```python
from build123d import *

# Parameters (mm, degrees)
SKETCH1_R           = 30
SKETCH1_R_2         = 21
BOSS_EXTRUDE1_DEPTH = 14
SKETCH1_3_R         = 32.5
SKETCH1_3_R_2       = 30
SKETCH1_3_R_3       = 21
BOSS_EXTRUDE2_DEPTH = 42
CUT_EXTRUDE1_START  = 14
SKETCH1_4_R         = 32.5
SKETCH1_4_R_2       = 30
CUT_EXTRUDE1_DEPTH  = 3
CHAMFER2_SIZE       = 2


with BuildPart() as part:
    # Sketch1 → Boss-Extrude1 (new body)
    # profile 1 of 8: a face of its own
    with BuildSketch(Plane(origin=(0, 0, 0), x_dir=(1, 0, 0), z_dir=(0, 1, 0))):
        Polygon((-18.763883749, -32.5), (18.763883749, -32.5), (37.527767497, 0), (18.763883749, 32.5), (-18.763883749, 32.5), (-37.527767497, 0), align=None)
        Circle(SKETCH1_R, mode=Mode.SUBTRACT)
    # profile 2 of 8: a face of its own
    with BuildSketch(Plane(origin=(0, 0, 0), x_dir=(1, 0, 0), z_dir=(0, 1, 0))):
        Circle(SKETCH1_R)
        with Locations(Location((0, 0, 0), (0, 0, 270))):
            Circle(SKETCH1_R_2, mode=Mode.SUBTRACT)
    # profile 3 of 8: a face of its own
    with BuildSketch(Plane(origin=(0, 0, 0), x_dir=(1, 0, 0), z_dir=(0, 1, 0))):
        with BuildLine():
            ThreePointArc((-5.3e-08, 32.5), (16.250000065, 28.145825585), (28.145825725, 16.249999824))
            Line((28.145825725, 16.249999824), (18.763883749, 32.5))
            Line((18.763883749, 32.5), (-5.3e-08, 32.5))
        make_face()
    # profile 4 of 8: a face of its own
    with BuildSketch(Plane(origin=(0, 0, 0), x_dir=(1, 0, 0), z_dir=(0, 1, 0))):
        with BuildLine():
            ThreePointArc((-28.14582555, 16.250000126), (-16.24999996, 28.145825646), (-5.3e-08, 32.5))
            Line((-5.3e-08, 32.5), (-18.763883749, 32.5))
            Line((-18.763883749, 32.5), (-28.14582555, 16.250000126))
        make_face()
    # profile 5 of 8: a face of its own
    with BuildSketch(Plane(origin=(0, 0, 0), x_dir=(1, 0, 0), z_dir=(0, 1, 0))):
        with BuildLine():
            Line((28.145825318, -16.250000528), (37.527767497, 0))
            Line((37.527767497, 0), (28.145825725, 16.249999824))
            ThreePointArc((28.145825725, 16.249999824), (31.392589381, 8.411618868), (32.5, 0))
            ThreePointArc((32.5, 0), (31.392589275, -8.41161926), (28.145825318, -16.250000528))
        make_face()
    # profile 6 of 8: a face of its own
    with BuildSketch(Plane(origin=(0, 0, 0), x_dir=(1, 0, 0), z_dir=(0, 1, 0))):
        with BuildLine():
            Line((18.763883749, -32.5), (28.145825318, -16.250000528))
            ThreePointArc((28.145825318, -16.250000528), (16.249999715, -28.145825788), (-4.8e-08, -32.5))
            Line((-4.8e-08, -32.5), (18.763883749, -32.5))
        make_face()
    # profile 7 of 8: a face of its own
    with BuildSketch(Plane(origin=(0, 0, 0), x_dir=(1, 0, 0), z_dir=(0, 1, 0))):
        with BuildLine():
            Line((-18.763883749, -32.5), (-4.8e-08, -32.5))
            ThreePointArc((-4.8e-08, -32.5), (-16.250000055, -28.145825591), (-28.145825663, -16.249999931))
            Line((-28.145825663, -16.249999931), (-18.763883749, -32.5))
        make_face()
    # profile 8 of 8: a face of its own
    with BuildSketch(Plane(origin=(0, 0, 0), x_dir=(1, 0, 0), z_dir=(0, 1, 0))):
        with BuildLine():
            ThreePointArc((-28.145825663, -16.249999931), (-32.5, 1.12e-07), (-28.14582555, 16.250000126))
            Line((-28.14582555, 16.250000126), (-37.527767497, 0))
            Line((-37.527767497, 0), (-28.145825663, -16.249999931))
        make_face()
    extrude(amount=BOSS_EXTRUDE1_DEPTH)

    # Sketch1<3> → Boss-Extrude2 (add)
    # profile 1 of 2: a face of its own
    with BuildSketch(Plane(origin=(0, 0, 0), x_dir=(1, 0, 0), z_dir=(0, 1, 0))):
        with Locations(Location((0, 0, 0), (0, 0, 270))):
            Circle(SKETCH1_3_R)
        Circle(SKETCH1_3_R_2, mode=Mode.SUBTRACT)
    # profile 2 of 2: a face of its own
    with BuildSketch(Plane(origin=(0, 0, 0), x_dir=(1, 0, 0), z_dir=(0, 1, 0))):
        Circle(SKETCH1_3_R_2)
        with Locations(Location((0, 0, 0), (0, 0, 270))):
            Circle(SKETCH1_3_R_3, mode=Mode.SUBTRACT)
    extrude(amount=BOSS_EXTRUDE2_DEPTH)

    # Sketch1<4> → Cut-Extrude1 (cut)
    with BuildSketch(Plane(origin=(0, 0, 0), x_dir=(1, 0, 0), z_dir=(0, 1, 0)).offset(CUT_EXTRUDE1_START)):
        with Locations(Location((0, 0, 0), (0, 0, 90))):
            Circle(SKETCH1_4_R)
        with Locations(Location((0, 0, 0), (0, 0, 270))):
            Circle(SKETCH1_4_R_2, mode=Mode.SUBTRACT)
    extrude(amount=CUT_EXTRUDE1_DEPTH, mode=Mode.SUBTRACT)

    # Chamfer2
    chamfer2_edges = [part.edges().sort_by_distance(p)[0] for p in [
        (0, 42, -32.5),
    ]]
    chamfer(chamfer2_edges, length=CHAMFER2_SIZE)


solid = part.part
```
Part model, mm, in its own coordinate system. A direction names the side the tool comes from. Coordinates: 2 decimals unless noted, no trailing zeros. Order: outer loops, then holes, each group sorted by start corner. A loop starts at its lowest first (then second) coordinate and runs counter-clockwise, first axis right, second up. Notation, with made-up numbers: (68, 39.5) - (125, 39.5) arc R15 ccw to (125, 60.5) - close; hole circle Ø3 at (47, 2.25). An arc over 180 degrees is marked (long way). Return JSON: item names as keys, results as strings. Group by question number.
Item 1: Cut at C-C (y = 28.5). List the corners of the cut face in (x, z), plus the area to 3 significant figures.
Item 2: Pin check, flat tips, straight feed: pin 1 (12 mm diameter, centred on x = 29.5, y = 35.5, fed in from -Z); pin 2 (1.5 mm diameter, centred on y = 16, z = 11, fed in from +X); pin 3 (12 mm diameter, centred on y = 25.5, z = -5.5, fed in from -X); pin 4 (8 mm diameter, centred on y = 16.5, z = -0.5, fed in from -X). Stop position of each tip, or through.
Item 3: Cut at B-B (y = 5.5). List the corners of the cut face in (x, z).
Item 4: Which spindle directions (+Z, -Z, +X, -X, +Y, -Y) get a long thin tool onto all of the face, cutting with end or side? Do faces 1 (the face through (-7, 42, 20)), 2 (the face through (9.76, 28.34, 31)), 3 (the face through (28, 14, -12)). Say none if no direction does.
Item 5: Pull direction X, two halves, no side cores. Call faces 4 (the face through (-29.9, 41.87, -6.64)), 5 (the face through (16, 0, -15)), 6 (the face through (6.31, 20.71, 20.03)): pulls with the +X half, pulls with the -X half, needs draft (parallel to the pull), parting line crosses it, or undercut.
Item 6: Cut at A-A (x = 0). List the corners of the cut face in (y, z), plus the area to 3 significant figures.
Item 7: Drill centre lines: probe 1 along X at (y, z) = (10, 0); probe 2 along X at (y, z) = (29, 0); probe 3 along Z at (x, y) = (3.5, 19). Where is each one in solid material? Low to high. Write a range as from..to.
Check values:
{
 "1": {"outline": "circle Ø65 at (0, 0); hole circle Ø42 at (0, 0)", "area": "1,930 mm2"},
 "2": {"pin 1": "stops at z = -22.45", "pin 2": "stops at x = 28.19", "pin 3": "stops at x = -32.5", "pin 4": "stops at x = -37.53"},
 "3": {"outline": "(-37.53, 0) - (-18.76, -32.5) - (18.76, -32.5) - (37.53, 0) - (18.76, 32.5) - (-18.76, 32.5) - close; hole circle Ø42 at (0, 0)"},
 "4": {"face 1": "+Z, -Z, +X, -X, +Y", "face 2": "+Y", "face 3": "none"},
 "5": {"face 4": "parting line crosses it", "face 5": "needs draft", "face 6": "undercut"},
 "6": {"outline": "(0, -32.5) - (14, -32.5) - (14, -30) - (17, -30) - (17, -32.5) - (40, -32.5) - (42, -30.5) - (42, -21) - (0, -21) - close; (0, 21) - (42, 21) - (42, 30.5) - (40, 32.5) - (17, 32.5) - (17, 30) - (14, 30) - (14, 32.5) - (0, 32.5) - close", "area": "947 mm2"},
 "7": {"probe 1": "x = -37.53..-21, 21..37.53", "probe 2": "x = -32.5..-21, 21..32.5", "probe 3": "z = -32.31..-20.71, 20.71..32.31"}
}
